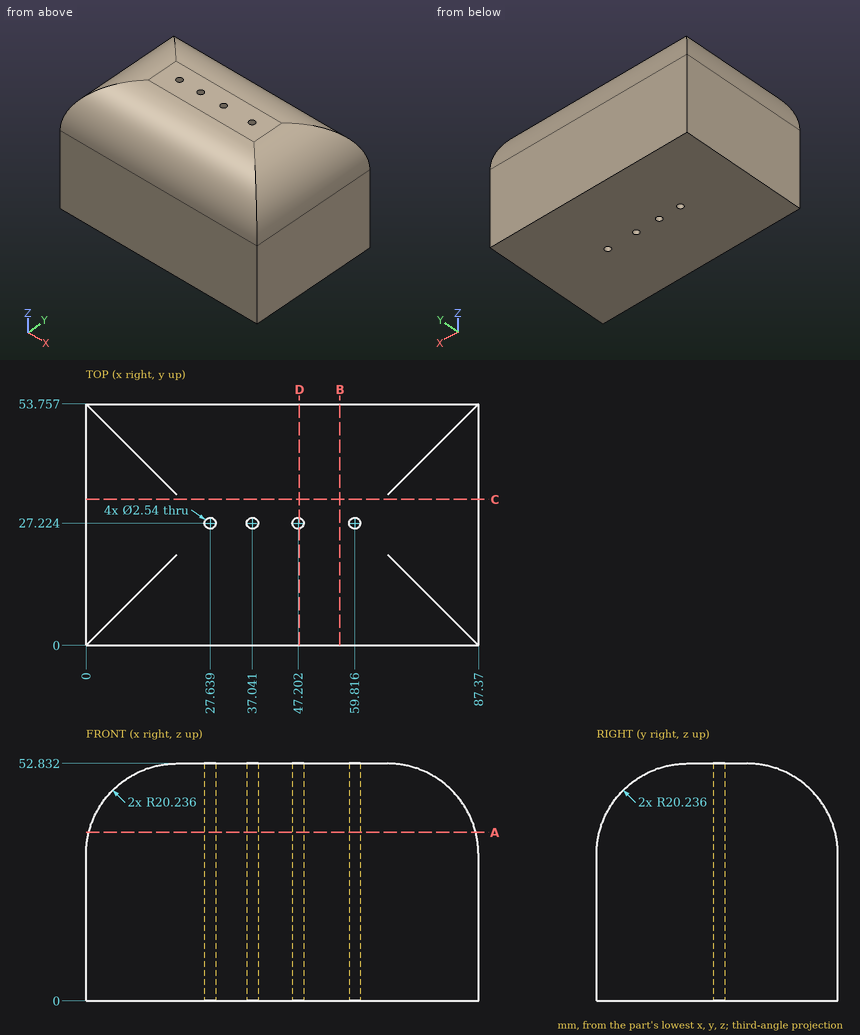
Study the drawing (mm; zero at the part's minimum x, y, z) and answer. Give positions to 0.01 mm unless a question says otherwise; leave off trailing zeros. Write each loop counter-clockwise with the first axis right and the second up, starting at its lowest first coordinate (ties: lowest second). Pieces come first, ordered by that corner, then holes. Notation, with made-up numbers: (47, 43) - (78, 43) arc R20 ccw to (78, 80) - close; hole circle Ø10 at (49, 14.25). An arc over 180 degrees is marked (long way). Use a Markdown table: item, result.
1. Section C-C on y = 32.5 is taken. Write down the section's boundary in (x, z) (1 decimal), plus the area to 3 significant figures.
Values follow:
| item | result |
|---|---|
| outline | (0, 0) - (87.4, 0) - (87.4, 32.6) arc R20.2 ccw to (67.1, 52.8) - (20.2, 52.8) arc R20.2 ccw to (0, 32.6) - close |
| area | 4,440 mm² |
2. Section B-B on x = 56.5 is taken. Write down the section's boundary in (y, z) (1 decimal), plus the area to 3 significant figures.
Values follow:
| item | result |
|---|---|
| outline | (0, 0) - (53.8, 0) - (53.8, 32.6) arc R20.2 ccw to (33.5, 52.8) - (20.2, 52.8) arc R20.2 ccw to (0, 32.6) - close |
| area | 2,660 mm² |
3. Find the intervals of material crossed by probe 1 along X at (y, z) = (27.5, 46) (1 decimal); probe 2 along Y at (x, z) = (27, 43) (1 decimal); probe 3 along Z at (x, y) = (31, 18), in increasing order. Write a range as from..to.
Values follow:
| item | result |
|---|---|
| probe 1 | x = 5.1..26.4, 28.9..35.8, 38.3..46, 48.4..58.6, 61.1..82.3 |
| probe 2 | y = 2.9..26.1, 28.3..50.9 |
| probe 3 | z = 0..52.71 |
4. Each of these flat-tipped pins is pushed along its axis until it touches: P1, Ø2, axis at x = 37.04, y = 27.22, coming from the -Z side; P2, Ø5, axis at x = 27.5, z = 36, coming from the +Y side; P3, Ø3, axis at y = 29, z = 47.5, coming from the -X side (1 decimal); P4, Ø4, axis at y = 10, z = 36, coming from the -X side. Where does it stop, or does it pass through?
Values follow:
| item | result |
|---|---|
| P1 | passes through |
| P2 | stops at y = 53.74 |
| P3 | stops at x = 5.1 |
| P4 | stops at x = 0.05 |
5. Section A-A on z = 37.5 is taken. Write down the section's boundary in (x, y) (1 decimal), plus the area to 3 significant figures.
Values follow:
| item | result |
|---|---|
| outline | (0.6, 0.6) - (86.8, 0.6) - (86.8, 53.2) - (0.6, 53.2) - close; hole circle Ø2.5 at (27.6, 27.2); hole circle Ø2.5 at (37, 27.2); hole circle Ø2.5 at (47.2, 27.2); hole circle Ø2.5 at (59.8, 27.2) |
| area | 4,510 mm² |
6. Section D-D on x = 47.5 is taken. Write down the section's boundary in (y, z) (1 decimal).
Values follow:
| item | result |
|---|---|
| outline | (0, 0) - (26, 0) - (26, 52.8) - (20.2, 52.8) arc R20.2 ccw to (0, 32.6) - close; (28.5, 0) - (53.8, 0) - (53.8, 32.6) arc R20.2 ccw to (33.5, 52.8) - (28.5, 52.8) - close |
